The drawing under review shows one solid part. Ordinate dimensions are in mm from its lowest x, y, z. A direction names the side the tool comes from. Coordinates: 2 decimals unless noted, no trailing zeros. Order: outer loops, then holes, each group sorted by start corner. A loop starts at its lowest first (then second) coordinate and runs counter-clockwise, first axis right, second up. Notation, with made-up numbers: (86.5, -15) - (138.5, -15) arc R11 ccw to (138.5, -6) - close; hole circle Ø4 at (-32.75, 68). An arc over 180 degrees is marked (long way). Answer in a Markdown table with one row per item.
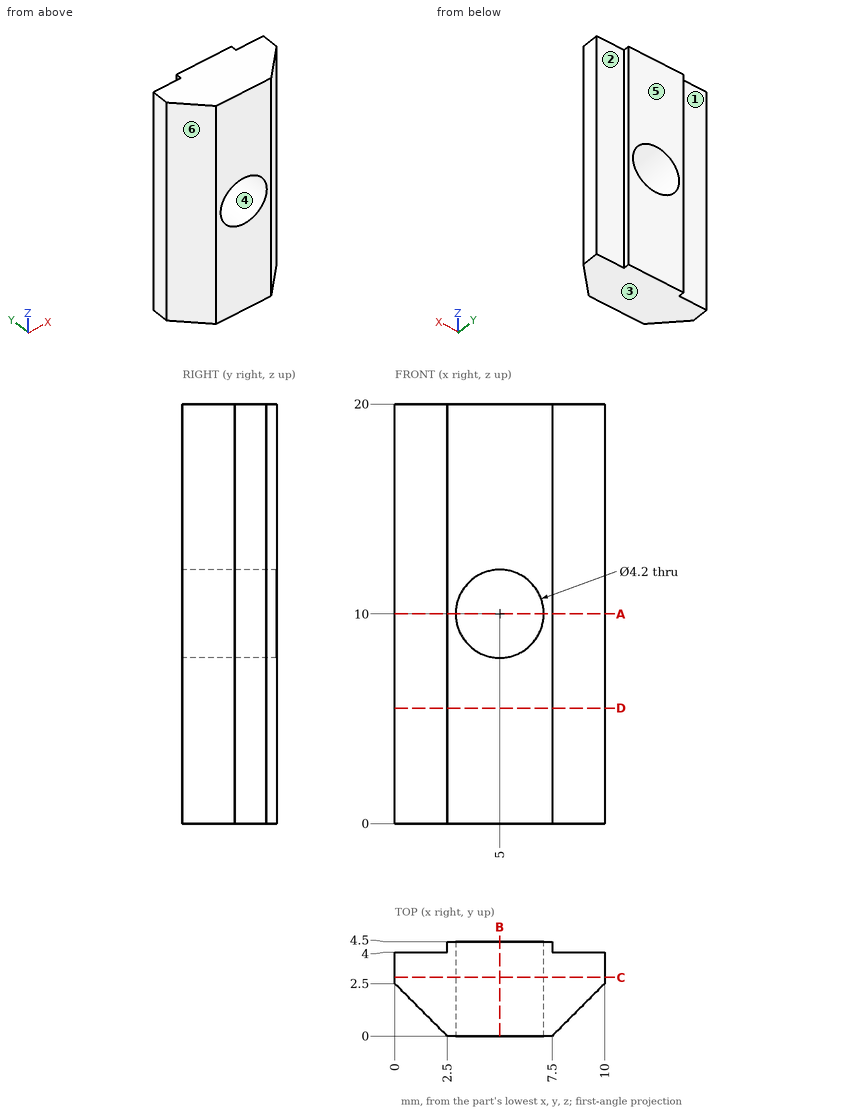
Item 1: Mouldability with a two-part tool opening along X and no side actions: class the marked faces 4, 5 and 6 as +X half, -X half, draft (parallel to the pull), parting line (faces both ways), or undercut.
Check values:
| item | result |
|---|---|
| face 4 | undercut |
| face 5 | draft |
| face 6 | -X half |
Item 2: We need section B-B, the plane x = 5. Write out the cut boundary in (y, z), then the cut area to 3 significant figures.
Check values:
| item | result |
|---|---|
| outline | (0, 0) - (4.5, 0) - (4.5, 7.9) - (0, 7.9) - close; (0, 12.1) - (4.5, 12.1) - (4.5, 20) - (0, 20) - close |
| area | 71.1 mm^2 |
Item 3: Clearance check with flat-ended pins moving along their axes: pin 1 Ø2.5 at (x, z) = (5, 10) entering from -Y; pin 2 Ø3 at (x, z) = (1.5, 14) entering from +Y; pin 3 Ø0.8 at (x, z) = (8.5, 11) entering from +Y. State where each tip first meets the part, or that it passes through.
Check values:
| item | result |
|---|---|
| pin 1 | through |
| pin 2 | y = 4.5 |
| pin 3 | y = 4 |
Item 4: We need section C-C, the plane y = 2.8. Write out the cut boundary in (x, z), then the cut area to 3 significant figures.
Check values:
| item | result |
|---|---|
| outline | (0, 0) - (10, 0) - (10, 20) - (0, 20) - close; hole circle Ø4.2 at (5, 10) |
| area | 186 mm^2 |
Item 5: We need section D-D, the plane z = 5.5. Write out the cut boundary in (x, y).
Check values:
| item | result |
|---|---|
| outline | (0, 2.5) - (2.5, 0) - (7.5, 0) - (10, 2.5) - (10, 4) - (7.5, 4) - (7.5, 4.5) - (2.5, 4.5) - (2.5, 4) - (0, 4) - close |
Item 6: We need section A-A, the plane z = 10. Write out the cut boundary in (x, y).
Check values:
| item | result |
|---|---|
| outline | (0, 2.5) - (2.5, 0) - (2.9, 0) - (2.9, 4.5) - (2.5, 4.5) - (2.5, 4) - (0, 4) - close; (7.1, 0) - (7.5, 0) - (10, 2.5) - (10, 4) - (7.5, 4) - (7.5, 4.5) - (7.1, 4.5) - close |
Item 7: Tool access review of the marked faces 1, 2 and 3: name each direction out of +Z, -Z, +X, -X, +Y, -Y from which nothing blocks a thin tool from reaching the whole face with its end or side.
Check values:
| item | result |
|---|---|
| face 1 | +Z, -Z, -X, +Y |
| face 2 | +Z, -Z, +X, +Y |
| face 3 | -Z, +X, -X, +Y, -Y |
Item 8: To check wall thickness, follow line 1 (X direction, y = 0.65, z = 9.75); line 2 (Z direction, x = 5, y = 2.05); line 3 (Z direction, x = 3.25, y = 1.8). State the ranges of each line that lie inside material, in increasing order. Write a range as from..to.
Check values:
| item | result |
|---|---|
| line 1 | 1.85..2.91, 7.09..8.15 |
| line 2 | 0..7.9, 12.1..20 |
| line 3 | 0..8.84, 11.16..20 |
